from build123d import *

# Parameters (mm, degrees)
SKETCH1_R           = 2.4892
BOSS_EXTRUDE1_DEPTH = 3.175
FILLET1_R           = 1.5875


with BuildPart() as part:
    # Sketch1 → Boss-Extrude1 (new, symmetric)
    with BuildSketch(Plane.XY):
        with BuildLine():
            Line((0, 27.3812), (69.85, 27.3812))
            Line((69.85, 27.3812), (69.85, -48.8188))
            Line((69.85, -48.8188), (25.42603388, -48.8188))
            Line((25.42603388, -48.8188), (25.42603388, -43.459816684))
            Line((25.42603388, -43.459816684), (40.915153964, -29.346022579))
            Line((40.915153964, -29.346022579), (18.162007104, -4.375683536))
            ThreePointArc((18.162007104, -4.375683536), (15.768494782, -0.923849067), (14.364087476, 3.034901057))
            ThreePointArc((14.364087476, 3.034901057), (9.246124703, 11.403806883), (0, 14.6812))
            Line((0, 14.6812), (0, 27.3812))
        make_face()
        with Locations((60.325, -23.4188)):
            Circle(SKETCH1_R, mode=Mode.SUBTRACT)
        with Locations((60.325, 14.6812)):
            Circle(SKETCH1_R, mode=Mode.SUBTRACT)
    extrude(amount=BOSS_EXTRUDE1_DEPTH, both=True)

    # Fillet1
    fillet1_edges = [part.edges().sort_by_distance(p)[0] for p in [
        (25.42603388, -43.459816684, 0),
        (40.915153964, -29.346022579, 0),
        (0, 14.6812, 0),
    ]]
    fillet(fillet1_edges, radius=FILLET1_R)


solid = part.part
Source: CAD feature listing. Evaluate the final solid. Frame: model axes, mm. A direction names the side the tool comes from. Coordinates: 2 decimals unless noted, no trailing zeros. Order: outer loops, then holes, each group sorted by start corner. A loop starts at its lowest first (then second) coordinate and runs counter-clockwise, first axis right, second up. Notation, with made-up numbers: M -35,64 L 15,64 A38 ccw 15,102 Z; hole C 16,50.5 d7. An arc over 180 degrees is marked long. Write each question's results on one line, items separated by ' | '. Start each with the question number.
Item 1: Cut plane D-D (x = 12.5). Return loops of the section in (y, z) (3 decimals), and give its area (3 significant figures).
Item 2: Cut plane B-B (z = 0.75). Count the separate pieces of the cut face and the enclosed holes in it, and give its area (3 significant figures).
Item 3: Line query: probe 1 along X at (y, z) = (16, 1.75); probe 2 along Y at (x, z) = (59, 2.5); probe 3 along X at (y, z) = (-22.5, 0.5). Output: solid intervals per line, ascending.
Item 4: Cut plane C-C (y = -40). Return loops of the section in (x, z) (3 decimals).
Item 5: Set-up query: faces 1 (the face through (25.426, -47, 0)), 2 (the face through (69.85, -10, 0)), 3 (the face through (29.156, -16.441, 0.044)). Return all of +Z, -Z, +X, -X, +Y, -Y with unobstructed straight access to the full face (end or side cutting, diameter ignored); none if empty.
Item 6: First-contact query: pin 1 Ø3.5 at (y, z) = (-46.5, -0.5) entering from -X; pin 2 Ø4.5 at (x, y) = (60.32, -23.42) entering from -Z. Flat tips, straight axial feed; report the tip coordinate or a pass-through.
Item 7: Draft query along X for faces 4 (the face through (32.746, -36.789, 0.044)), 5 (the face through (58.35, 13.167, -0.044)), 6 (the face through (43, -2, 3.175)), 7 (the face through (57.84, -23.31, -0.04)). Return one class per face: pulls with the +X half, pulls with the -X half, needs draft (parallel to the pull), parting line crosses it, or undercut.
Item 8: Cut plane A-A (x = 33). Return loops of the section in (y, z) (3 decimals).
Checked values:
1) outline: M 7.7,-3.175 L 27.381,-3.175 L 27.381,3.175 L 7.7,3.175 Z | area: 125 mm2
2) separate pieces: 1 | enclosed holes: 2 | area: 3,700 mm2
3) probe 1: x = 0.01 to 58.21, 62.44 to 69.85 | probe 2: y = -48.82 to -25.53, -21.31 to 12.57, 16.79 to 27.38 | probe 3: x = 34.68 to 58.01, 62.64 to 69.85
4) outline: M 29.223,-3.175 L 69.85,-3.175 L 69.85,3.175 L 29.223,3.175 Z
5) face 1: +Z, -Z, -X, -Y | face 2: +Z, -Z, +X, +Y, -Y | face 3: +Z, -Z, -X
6) pin 1: stops at x = 25.43 | pin 2: passes through
7) face 4: pulls with the -X half | face 5: undercut | face 6: needs draft | face 7: undercut
8) outline: M -48.819,-3.175 L -36.558,-3.175 L -36.558,3.175 L -48.819,3.175 Z; M -20.66,-3.175 L 27.381,-3.175 L 27.381,3.175 L -20.66,3.175 Z
